Autodesk Inventor part; units mm, degrees
ref_plane "YZ Plane" through (0, 0, 0) normal (1, 0, 0) x (0, 1, 0)
ref_plane "XZ Plane" through (0, 0, 0) normal (0, 1, 0) x (-1, 0, 0)
ref_plane "XY Plane" through (0, 0, 0) normal (0, 0, 1) x (1, 0, 0)
sketch "Sketch1" plane through (0, 0, 0) normal (0, 0, 1) x (1, 0, 0)
  line L0 (-175, 0) -> (175, 0)
  line L1 (0, -140) -> (0, 140)
  line L2 (-125, 100) -> (125, 100)
  line L3 (125, 100) -> (125, -100)
  line L4 (125, -100) -> (-125, -100)
  line L5 (-125, -100) -> (-125, 100)
  point P0 (0, 0)
  dimension "d0" = 200
  dimension "d1" = 250
extrude "Extrusion1" add sketch "Sketch1" against normal blind 180
fillet "Fillet5" radius 80 2 edges at (0, -100, 0) (0, 100, 0)
fillet "Fillet6" radius 65 10 edges at (125, 0, 0) (125, 76.5685, -23.4315) (125, 100, -130) (125, -100, -130) (125, -76.5685, -23.4315) (-125, -100, -130) (-125, 0, 0) (-125, 76.5685, -23.4315) (-125, 100, -130) (-125, -76.5685, -23.4315)
shell "Shell1" thickness 5 removed faces 1 at (20, -33.3333, -180)
sketch "Sketch5" plane through (-60, -100, -180) normal (0, -1, 0) x (1, 0, 0)
  line L0 (120, 0) -> (120, 100)
  line L1 (70, 96.5308) -> (120, 96.5308)
  line L2 (120, 96.5308) -> (120, 71.5308)
  line L3 (120, 71.5308) -> (70, 71.5308)
  line L4 (70, 71.5308) -> (70, 96.5308)
  point P0 (60, 180)
  dimension "d15" = 25
  dimension "d16" = 50
extrude "Extrusion3" cut sketch "Sketch5" against normal blind 24
sketch "Sketch6" plane through (-60, -100, -80) normal (0, -1, 0) x (1, 0, 0)
  circle A0 centre (55, -15.7839) radius 7.5
  line L0 (70, -28.4692) -> (70, -3.4692)
  point P0 (60, 80)
  point P1 (70, -15.9692)
  dimension "d19" = 15
  dimension "d20" = 15
extrude "Extrusion4" add sketch "Sketch6" along normal blind 25
sketch "Sketch7" plane through (-60, -100, -80) normal (0, -1, 0) x (1, 0, 0)
  circle A0 centre (95, -60.7349) radius 11
  line L0 (120, -28.4692) -> (120, -100)
  point P0 (60, 80)
  dimension "d23" = 25
  dimension "d24" = 22
extrude "Extrusion5" add sketch "Sketch7" along normal blind 20
fillet "Fillet7" radius 1.5 1 edges at (-12.5, -125, -95.7839)
fillet "Fillet8" radius 1.5 1 edges at (24, -120, -140.7349)
sketch "Sketch8" plane through (-60, -95, -180) normal (0, 1, 0) x (1, 0, 0)
  line L0 (120, -96.5308) -> (70, -96.5308)
  line L1 (70, -96.5308) -> (70, -71.5308)
  line L2 (70, -71.5308) -> (120, -71.5308)
  line L3 (120, -71.5308) -> (120, 0)
  line L4 (0, 0) -> (120, 0)
  line L5 (0, 0) -> (0, -100)
  line L6 (0, -100) -> (120, -100)
  line L7 (120, -100) -> (120, -96.5308)
  line L8 (103.331, -9.0858) -> (93.331, -9.0858)
  line L9 (93.331, -9.0858) -> (93.331, -12.0858)
  line L10 (93.331, -12.0858) -> (103.331, -12.0858)
  line L11 (103.331, -12.0858) -> (103.331, -9.0858)
  line L12 (60, -9.0858) -> (50, -9.0858)
  line L13 (50, -9.0858) -> (50, -12.0858)
  line L14 (50, -12.0858) -> (60, -12.0858)
  line L15 (60, -12.0858) -> (60, -9.0858)
  point P0 (60, -180)
  dimension "d29" = 10
  dimension "d30" = 3
  dimension "d31" = 10
extrude "Extrusion6" add sketch "Sketch8" along normal blind 15 contours L11 L10 L9 L8 | L15 L14 L13 L12
sketch "Sketch9" plane through (-10, -95, -167.9142) normal (0, 0, 1) x (1, 0, 0)
  line L0 (0, 0) -> (0, 15)
  line L1 (10, 0) -> (10, 15)
  line L2 (0, 9.5743) -> (10, 9.5743)
  line L3 (10, 9.5743) -> (10, 15)
  line L4 (10, 15) -> (0, 15)
  line L5 (0, 15) -> (0, 9.5743)
  line L6 (53.331, 15) -> (43.331, 15)
  line L7 (43.2725, 9.5743) -> (53.331, 9.5743)
  line L8 (53.331, 9.5743) -> (53.331, 15)
  line L9 (53.331, 15) -> (43.2725, 15)
  line L10 (43.2725, 15) -> (43.2725, 9.5743)
  point P0 (10, 95)
extrude "Extrusion7" add sketch "Sketch9" along normal blind 5
sketch "Sketch10" plane through (125, -35, -180) normal (1, 0, 0) x (0, 0, -1)
  line L0 (0, 0) -> (-100, 0)
  line L1 (0, 70) -> (0, 0)
  line L2 (-100, 70) -> (0, 70)
  arc A0 (-100, 70) -> (-115, 55) centre (-100, 55) ccw
  line L3 (-115, 15) -> (-115, 55)
  arc A1 (-115, 15) -> (-100, 0) centre (-100, 15) ccw
  circle A2 centre (-47.024, 35) radius 12.5
  point P0 (-180, 35)
  dimension "d36" = 25
extrude "Extrusion8" cut sketch "Sketch10" against normal blind 25 contours A2
sketch "Sketch11" plane through (-60, 100, -80) normal (0, 1, 0) x (1, 0, 0)
  line L0 (40, 60) -> (10, 60)
  line L1 (10, 60) -> (10, 80)
  line L2 (10, 80) -> (40, 80)
  line L3 (40, 80) -> (40, 60)
  line L4 (0, 0) -> (0, 100)
  line L5 (0, 100) -> (120, 100)
  point P0 (60, -80)
  point P1 (10, 70)
  dimension "d41" = 30
  dimension "d42" = 20
  dimension "d43" = 10
  dimension "d44" = 20
extrude "Extrusion9" cut sketch "Sketch11" against normal blind 10
sketch "Sketch12" plane through (-60, 100, -80) normal (0, 1, 0) x (1, 0, 0)
  line L0 (70, 65) -> (50, 65)
  line L1 (50, 65) -> (50, 80)
  line L2 (50, 80) -> (70, 80)
  line L3 (70, 80) -> (70, 65)
  line L4 (40, 80) -> (40, 60)
  line L5 (0, 100) -> (120, 100)
  point P0 (60, -80)
  dimension "d47" = 10
  dimension "d48" = 20
  dimension "d49" = 15
  dimension "d50" = 20
extrude "Extrusion10" cut sketch "Sketch12" against normal blind 10
sketch "Sketch13" plane through (0, 0, -180) normal (0, 0, -1) x (-1, 0, 0)
  arc A0 (-60, 95) -> (-120, 35) centre (-60, 35) ccw
  line L0 (-60, 95) -> (60, 95)
  arc A1 (120, 35) -> (60, 95) centre (60, 35) ccw
  line L1 (120, 35) -> (120, -35)
  arc A2 (60, -95) -> (120, -35) centre (60, -35) ccw
  line L2 (60, -95) -> (-60, -95)
  arc A3 (-120, -35) -> (-60, -95) centre (-60, -35) ccw
  line L3 (-120, -35) -> (-120, 35)
  arc A4 (125, 35) -> (60, 100) centre (60, 35) ccw
  line L4 (60, 100) -> (-60, 100)
  arc A5 (-60, 100) -> (-125, 35) centre (-60, 35) ccw
  line L5 (-125, 35) -> (-125, -35)
  arc A6 (-125, -35) -> (-60, -100) centre (-60, -35) ccw
  line L6 (-60, -100) -> (60, -100)
  arc A7 (60, -100) -> (125, -35) centre (60, -35) ccw
  line L7 (125, -35) -> (125, 35)
  line L8 (193.8467, 0) -> (-193.8467, 0)
  line L9 (0, -172.6924) -> (0, 161.1543)
  point P0 (0, 0)
extrude "Extrusion11" add sketch "Sketch13" along normal blind 5
properties part number "Protosaber Case"
Source: CAD feature listing. Evaluate the final solid. Frame: model axes, mm. A direction names the side the tool comes from. Coordinates: 2 decimals unless noted, no trailing zeros. Write each loop counter-clockwise with the first axis right and the second up, starting at its lowest first coordinate (ties: lowest second). Pieces come first, ordered by that corner, then holes. Notation, with made-up numbers: M 68,-21 L 100,-21 A19 ccw 100,6 Z; hole C 43,46.5 d3. An arc over 180 degrees is marked long. Use a Markdown table: item, result.
1) Ray query, L1, parallel to Y at x = 60, z = -118; L2, parallel to X at y = -17.5, z = -103; L3, parallel to Z at x = 1, y = -39.5. Return the intervals inside material, ascending.
Conclusion:
| item | result |
|---|---|
| L1 | y = -100 to -95, 95 to 100 |
| L2 | x = -125 to -120, 120 to 125 |
| L3 | z = -185 to -180, -7.58 to -2.41 |
2) Reachability of faces 1 (the cylindrical face through (0.84, -72.45, -26.39)), 2 (the cylindrical face through (105.454, -81.465, -131.765)) from +Z, -Z, +X, -X, +Y, -Y: full face, straight path, thin tool, end or side. Return the list, or none.
Conclusion:
| item | result |
|---|---|
| face 1 | none |
| face 2 | +Z, -Z, +X, -Y |
3) Mould query, pull axis Z, two halves, no side actions, for faces 3 (the cylindrical face through (32.6, -109.1, -130)), 4 (the flat face through (38, -88, -170.914)), 5 (the flat face through (125, 0, -111)), 6 (the cylindrical face through (0.84, 77.19, -24.06)). Classes: pulls with the +Z half, pulls with the -Z half, needs draft (parallel to the pull), parting line crosses it, or undercut.
Conclusion:
| item | result |
|---|---|
| face 3 | parting line crosses it |
| face 4 | undercut |
| face 5 | needs draft |
| face 6 | pulls with the +Z half |
4) Section B-B, the plane x = -5. Output: boundary loops of the cut face in (y, z), then the cut area to 3 significant figures.
Conclusion:
| item | result |
|---|---|
| outline | M -125,-101.78 A1.5 ccw -123.5,-103.28 L -100,-103.28 L -100,-185 L 100,-185 L 100,-160 L 95,-160 L 95,-180 L -95,-180 L -95,-170.91 L -80,-170.91 L -80,-162.91 L -85.43,-162.91 L -85.43,-167.91 L -95,-167.91 L -95,-80 A75 cw -20,-5 L 20,-5 A75 cw 95,-80 L 95,-145 L 100,-145 L 100,-80 A80 ccw 20,0 L -20,0 A80 ccw -100,-80 L -100,-88.28 L -123.5,-88.28 A1.5 ccw -125,-89.78 Z |
| area | 3,790 mm^2 |
5) First-contact query: pin 1 Ø5.5 at (x, z) = (31.5, -140) entering from -Y; pin 2 Ø2.5 at (y, z) = (-89, -169) entering from -X; pin 3 Ø3 at (y, z) = (-8, -35.5) entering from -X. Flat tips, straight axial feed; report the tip coordinate or a pass-through.
Conclusion:
| item | result |
|---|---|
| pin 1 | stops at y = -120 |
| pin 2 | stops at x = -97.98 |
| pin 3 | stops at x = -118.66 |
6) Section A-A, the plane y = 0. Output: boundary loops of the cut face in (x, z).
Conclusion:
| item | result |
|---|---|
| outline | M -125,-185 L 125,-185 L 125,-145.48 L 120,-145.48 L 120,-180 L -120,-180 L -120,-65 A60 cw -60,-5 L 60,-5 A60 cw 120,-65 L 120,-120.48 L 125,-120.48 L 125,-65 A65 ccw 60,0 L -60,0 A65 ccw -125,-65 Z |
